Part print with two shaded views. Sizes in mm from the minimum x, y, z corner. A direction names the side the tool comes from. Coordinates: 2 decimals unless noted, no trailing zeros. Order: outer loops, then holes, each group sorted by start corner. A loop starts at its lowest first (then second) coordinate and runs counter-clockwise, first axis right, second up. Notation, with made-up numbers: (-33, 12.5) - (8, 12.5) arc R14 cw to (8, 20.5) - close; hole circle Ø6 at (79, 88.5). An arc over 180 degrees is marked (long way). Write each question's results on one line, items separated by ' | '. Start each with the question number.
Q1. Band-saw the part on A-A, the plane x = 38. Write the cut outline in (y, z).
Q2. Band-saw the part on D-D, the plane y = 29. Write the cut outline in (x, z) (1 decimal).
Q3. Pin check, flat tips, straight feed: P1, Ø1, axis at x = 10.5, y = 25, coming from the +Z side; P2, Ø6, axis at x = 39, y = 33.5, coming from the -Z side; P3, Ø10, axis at y = 26, z = 24.5, coming from the -X side; P4, Ø2, axis at x = 47, y = 12, coming from the +Z side. Stop position of each tip, or through.
Q4. Band-saw the part on C-C, the plane y = 20.5. Write the cut outline in (x, z), then the cut area to 3 significant figures.
Q5. Which spindle directions (+Z, -Z, +X, -X, +Y, -Y) get a long thin tool onto all of the face, cutting with end or side? Do the marked faces 1 and 2. Say none if no direction does.
Q6. Pull direction X, two halves, no side cores. Call the marked faces 3, 4 and 5: released by +X, released by -X, zero draft, split by the parting line, or undercut.
Q7. Band-saw the part on B-B, the plane y = 10. Write the cut outline in (x, z), then the cut area to 3 significant figures.
Q8. Wall check: probe 1 along X at (y, z) = (22, 38); probe 2 along Z at (x, y) = (49.5, 8); probe 3 along Y at (x, z) = (38.5, 68.5). Give the ranges that are in metal, low to high.
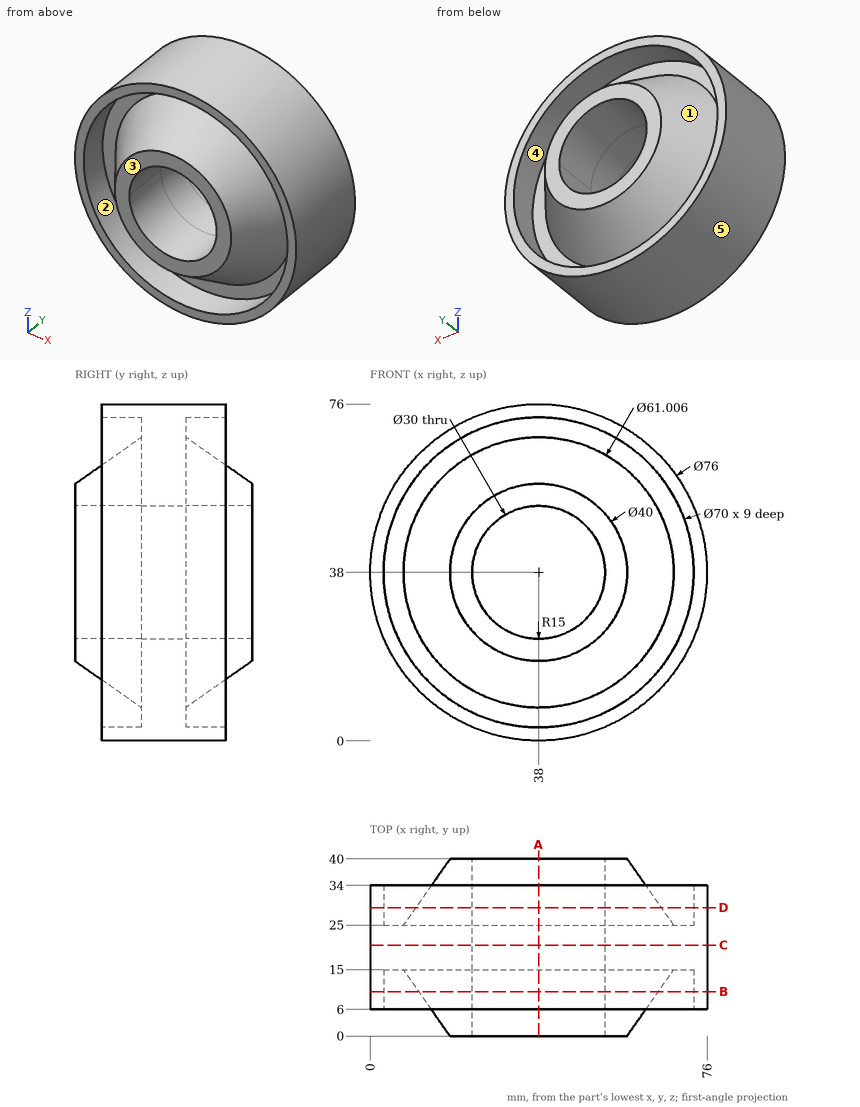
Results below:
1) outline: (0, 18) - (15, 7.5) - (15, 3) - (6, 3) - (6, 0) - (34, 0) - (34, 3) - (25, 3) - (25, 7.5) - (40, 18) - (40, 23) - (0, 23) - close; (0, 53) - (40, 53) - (40, 58) - (25, 68.5) - (25, 73) - (34, 73) - (34, 76) - (6, 76) - (6, 73) - (15, 73) - (15, 68.5) - (0, 58) - close
2) outline: circle Ø76 at (38, 38); circle Ø55.4 at (38, 38); hole circle Ø70 at (38, 38); hole circle Ø30 at (38, 38)
3) P1: stops at z = 64.74 | P2: stops at z = 0 | P3: stops at x = 0.96 | P4: stops at z = 75.15
4) outline: circle Ø76 at (38, 38); hole circle Ø30 at (38, 38) | area: 3,830 mm²
5) face 1: +Y | face 2: -Y
6) face 3: zero draft | face 4: undercut | face 5: split by the parting line
7) outline: circle Ø76 at (38, 38); circle Ø54 at (38, 38); hole circle Ø70 at (38, 38); hole circle Ø30 at (38, 38) | area: 2,270 mm²
8) probe 1: x = 0 to 23, 53 to 76 | probe 2: z = 1.78 to 4.94, 15.13 to 28.37, 47.63 to 60.87, 71.06 to 74.22 | probe 3: y = 15 to 25
